```python
from build123d import *

# Parameters (mm, degrees)
SKETCH_1_R          = 28
SKETCH_1_R_2        = 14
EXTRUDE_1_DEPTH     = 6
CUT_EXTRUDE_START   = 4.5
SKETCH_1_4_R        = 20
SKETCH_1_4_R_2      = 14
CUT_EXTRUDE_1_DEPTH = 1.5
M3X0_5_1_D          = 2.5
HOLE_WIZARD_M3_1_D  = 3.2


with BuildPart() as part:
    # ｽｹｯﾁ1 → ﾎﾞｽ - 押し出し1 (new body)
    with BuildSketch(Plane.XY):
        Circle(SKETCH_1_R)
        Circle(SKETCH_1_R_2, mode=Mode.SUBTRACT)
    extrude(amount=EXTRUDE_1_DEPTH)

    # ｽｹｯﾁ1<4> → ｶｯﾄ - 押し出し1 (cut)
    with BuildSketch(Plane.XY.offset(CUT_EXTRUDE_START)):
        Circle(SKETCH_1_4_R)
        Circle(SKETCH_1_4_R_2, mode=Mode.SUBTRACT)
    extrude(amount=CUT_EXTRUDE_1_DEPTH, mode=Mode.SUBTRACT)

    # M3x0.5 ねじ穴用ねじ下穴ﾄﾞﾘﾙ1 (through all)
    with Locations(Plane(origin=(17.5, 0, 0), x_dir=(-1, 0, 0), z_dir=(0, 0, -1))):
        with Locations((0, 0), (8.75, -15.155444566), (26.25, -15.155444566), (35, 0), (26.25, 15.155444566), (8.75, 15.155444566)):
            Hole(M3X0_5_1_D / 2)

    # M3 すきま穴1 (through all)
    with Locations(Plane(origin=(0, 25, 0), x_dir=(-1, 0, 0), z_dir=(0, 0, -1))):
        with Locations((0, 0), (-17.67766953, -7.32233047), (-25, -25), (-17.67766953, -42.67766953), (0, -50), (17.67766953, -42.67766953), (25, -25), (17.67766953, -7.32233047)):
            Hole(HOLE_WIZARD_M3_1_D / 2)


solid = part.part
```
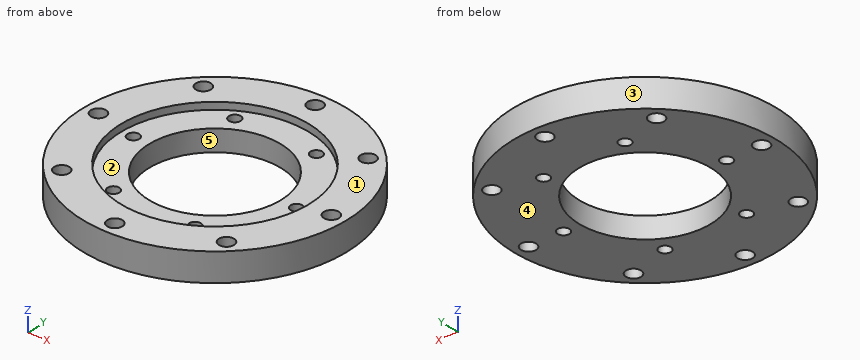
Build history of the part. All positions in model axes, mm. Face numbers are marked on the shaded views. A direction names the side the tool comes from. Give positions to 0.01 mm unless a question says otherwise; leave off trailing zeros. Loops run counter-clockwise (first coordinate to the right, second up) from the corner with the lowest first, then second, coordinate; pieces in that order, holes last.
Item 1: Slice it at C-C, the plane x = 11. List the corners of the cut face in (y, z).
Answers follow:
outline: (-25.75, 0) - (-8.66, 0) - (-8.66, 4.5) - (-16.7, 4.5) - (-16.7, 6) - (-25.75, 6) - close; (8.66, 0) - (25.75, 0) - (25.75, 6) - (16.7, 6) - (16.7, 4.5) - (8.66, 4.5) - close
Item 2: Flat gauge pins, fed straight in: pin 1 (2 mm diameter, centred on x = 18.5, y = 0, fed in from +Z); pin 2 (2 mm diameter, centred on x = 13, z = 5, fed in from -Y); pin 3 (2 mm diameter, centred on y = 10.5, z = 3, fed in from -X). Where does each tip first touch, or does it go through?
Answers follow:
pin 1: stops at z = 4.5
pin 2: stops at y = -25.3
pin 3: stops at x = -26.34
Item 3: Slice it at A-A, the plane x = 0. List the corners of the cut face in (y, z).
Answers follow:
outline: (-28, 0) - (-26.6, 0) - (-26.6, 6) - (-28, 6) - close; (-23.4, 0) - (-14, 0) - (-14, 4.5) - (-20, 4.5) - (-20, 6) - (-23.4, 6) - close; (14, 0) - (23.4, 0) - (23.4, 6) - (20, 6) - (20, 4.5) - (14, 4.5) - close; (26.6, 0) - (28, 0) - (28, 6) - (26.6, 6) - close
Item 4: Slice it at D-D, the plane y = -25. List the corners of the cut face in (x, z).
Answers follow:
outline: (-12.61, 0) - (-1.6, 0) - (-1.6, 6) - (-12.61, 6) - close; (1.6, 0) - (12.61, 0) - (12.61, 6) - (1.6, 6) - close
Item 5: Drill centre lines: line 1 (Y direction, x = 0, z = 4.9); line 2 (Y direction, x = 8.75, z = 2.05); line 3 (X direction, y = -17, z = 0.7). Where is each one in solid material? Low to high.
Answers follow:
line 1: y = -28 to -26.6, -23.4 to -20, 20 to 23.4, 26.6 to 28
line 2: y = -26.6 to -16.41, -13.91 to -10.93, 10.93 to 13.91, 16.41 to 26.6
line 3: x = -22.25 to -19.13, -16.23 to 16.23, 19.13 to 22.25
Item 6: Which spindle directions (+Z, -Z, +X, -X, +Y, -Y) get a long thin tool onto all of the face, cutting with end or side? Do the marked faces 1 and 2. Say none if no direction does.
Answers follow:
face 1: +Z, +X, -X, +Y, -Y
face 2: +Z
Item 7: Slice it at B-B, the plane y = -18.5. List the corners of the cut face in (x, z).
Answers follow:
outline: (-21.02, 0) - (-19.05, 0) - (-19.05, 6) - (-21.02, 6) - close; (-16.31, 0) - (16.31, 0) - (16.31, 6) - (7.6, 6) - (7.6, 4.5) - (-7.6, 4.5) - (-7.6, 6) - (-16.31, 6) - close; (19.05, 0) - (21.02, 0) - (21.02, 6) - (19.05, 6) - close
Item 8: Pull direction X, two halves, no side cores. Call the marked faces 3, 4 and 5: released by +X, released by -X, zero draft, split by the parting line, or undercut.
Answers follow:
face 3: split by the parting line
face 4: zero draft
face 5: undercut
